Build history of the part. All positions in model axes, mm. Face numbers are marked on the shaded views. A direction names the side the tool comes from. Round coordinates to 2 decimals unless told otherwise and drop trailing zeros. Loops run counter-clockwise (first coordinate to the right, second up) from the corner with the lowest first, then second, coordinate; pieces in that order, holes last. Notation, with made-up numbers: (-34.5, 64.5) - (-30.5, 64.5) arc R33 cw to (-30.5, 96.5) - close; hole circle Ø7 at (37, 87.5). An arc over 180 degrees is marked (long way). Use one line per item in the form item = value. Start each with the question number.
Q1. Saw through at C-C (x = 4.25). Give the cut face in (y, z).
Q2. Drill centre lines: line 1 (Y direction, x = -1.1, z = 12.3); line 2 (X direction, y = 2, z = 5.5); line 3 (X direction, y = 4, z = -1.75). Where is each one in solid material? Low to high.
Q3. Pin check, flat tips, straight feed: pin 1 (3 mm diameter, centred on x = -1.1, y = 5, fed in from +Z); pin 2 (1.2 mm diameter, centred on x = -1.1, y = 11.75, fed in from +Z); pin 3 (2 mm diameter, centred on x = -9, z = 1.5, fed in from +Y). Stop position of each tip, or through.
Q4. 3-axis set-ups, long thin cutter, end or side, ignore diameter. For the marked faces 4 and 5: which of +Z, -Z, +X, -X, +Y, -Y reach the whole face in a straight line?
Q5. Saw through at B-B (z = 2.25). Give the cut face in (x, y).
Q6. Saw through at D-D (y = 5). Give the cut face in (x, z).
Q7. Saw through at A-A (y = 7). Give the cut face in (x, z).
Q8. Mould opens along Z. For the marked faces 1, 2 and 3 say: released by +Z, released by -Z, zero draft, split by the parting line, or undercut.
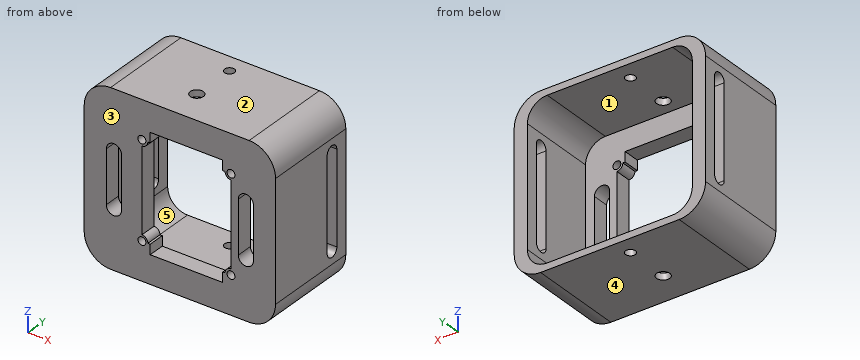
```python
from build123d import *

# Parameters (mm, degrees)
SKETCH1_W                = 25
SKETCH1_H                = 24
SKETCH1_R                = 0.6
BOSS_EXTRUDE1_DEPTH      = 2.5
CUT_EXTRUDE1_DEPTH       = 3.5
SKETCH8_W                = 11
SKETCH8_H                = 17.5
CUT_EXTRUDE4_DEPTH       = 3.5
SKETCH2_W                = 29
SKETCH2_H                = 26
SKETCH2_W_2              = 25
SKETCH2_H_2              = 24
BOSS_EXTRUDE2_DEPTH      = 12
BOSS_EXTRUDE2_DEPTH_BACK = 2.5
SKETCH5_R                = 0.75
SKETCH5_R_2              = 1
CUT_EXTRUDE2_DEPTH       = 26
CUT_EXTRUDE2_DEPTH_BACK  = 2
FILLET1_R                = 3
FILLET2_R                = 4
CUT_EXTRUDE5_DEPTH       = 30


with BuildPart() as part:
    # Sketch1 → Boss-Extrude1 (new body)
    with BuildSketch(Plane(origin=(0, 0, 0), x_dir=(1, 0, 0), z_dir=(0, 1, 0))):
        Rectangle(SKETCH1_W, SKETCH1_H)
        with Locations((7.75, 7.25)):
            Circle(SKETCH1_R, mode=Mode.SUBTRACT)
        with Locations((7.75, -7.25)):
            Circle(SKETCH1_R, mode=Mode.SUBTRACT)
        with Locations((-5.75, -7.25)):
            Circle(SKETCH1_R, mode=Mode.SUBTRACT)
        with Locations((-5.75, 7.25)):
            Circle(SKETCH1_R, mode=Mode.SUBTRACT)
        with BuildLine():
            Line((8.85, -4), (8.85, 4))
            ThreePointArc((8.85, 4), (10, 5.15), (11.15, 4))
            Line((11.15, 4), (11.15, -4))
            ThreePointArc((11.15, -4), (10, -5.15), (8.85, -4))
        make_face(mode=Mode.SUBTRACT)
        with BuildLine():
            Line((-8.85, -4), (-8.85, 4))
            ThreePointArc((-8.85, 4), (-10, 5.15), (-11.15, 4))
            Line((-11.15, 4), (-11.15, -4))
            ThreePointArc((-11.15, -4), (-10, -5.15), (-8.85, -4))
        make_face(mode=Mode.SUBTRACT)
    extrude(amount=BOSS_EXTRUDE1_DEPTH)

    # Sketch3 → Cut-Extrude1 (cut, through all)
    with BuildSketch(Plane(origin=(0, 2.5, 0), x_dir=(1, 0, 0), z_dir=(0, 1, 0))):
        with BuildLine():
            Line((-4.85, 7.25), (6.85, 7.25))
            ThreePointArc((6.85, 7.25), (7.113603897, 6.613603897), (7.75, 6.35))
            Line((7.75, 6.35), (7.75, -6.35))
            ThreePointArc((7.75, -6.35), (7.113603897, -6.613603897), (6.85, -7.25))
            Line((6.85, -7.25), (-4.85, -7.25))
            ThreePointArc((-4.85, -7.25), (-5.113603897, -6.613603897), (-5.75, -6.35))
            Line((-5.75, -6.35), (-5.75, 6.35))
            ThreePointArc((-5.75, 6.35), (-5.113603897, 6.613603897), (-4.85, 7.25))
        make_face()
    extrude(amount=-CUT_EXTRUDE1_DEPTH, mode=Mode.SUBTRACT)

    # Sketch8 → Cut-Extrude4 (cut, through all)
    with BuildSketch(Plane(origin=(0, 2.5, 0), x_dir=(1, 0, 0), z_dir=(0, 1, 0))):
        with Locations((1, 0)):
            Rectangle(SKETCH8_W, SKETCH8_H)
    extrude(amount=-CUT_EXTRUDE4_DEPTH, mode=Mode.SUBTRACT)

    # Sketch2 → Boss-Extrude2 (add, two sides)
    with BuildSketch(Plane(origin=(0, 2.5, 0), x_dir=(1, 0, 0), z_dir=(0, 1, 0))) as boss_extrude2_sk:
        Rectangle(SKETCH2_W, SKETCH2_H)
        Rectangle(SKETCH2_W_2, SKETCH2_H_2, mode=Mode.SUBTRACT)
    extrude(amount=BOSS_EXTRUDE2_DEPTH)
    extrude(boss_extrude2_sk.sketch, amount=-BOSS_EXTRUDE2_DEPTH_BACK)

    # Sketch5 → Cut-Extrude2 (cut, two sides)
    with BuildSketch(Plane.XY.offset(-12)) as cut_extrude2_sk:
        with Locations((-1.1, 11.75)):
            Circle(SKETCH5_R)
        with Locations((-1.1, 5)):
            Circle(SKETCH5_R_2)
    extrude(amount=CUT_EXTRUDE2_DEPTH, mode=Mode.SUBTRACT)
    extrude(cut_extrude2_sk.sketch, amount=-CUT_EXTRUDE2_DEPTH_BACK, mode=Mode.SUBTRACT)

    # Fillet1
    fillet1_edges = [part.edges().sort_by_distance(p)[0] for p in [
        (12.5, 8.5, 12),
        (-12.5, 8.5, -12),
        (12.5, 8.5, -12),
        (-12.5, 8.5, 12),
    ]]
    fillet(fillet1_edges, radius=FILLET1_R)

    # Fillet2
    fillet2_edges = [part.edges().sort_by_distance(p)[0] for p in [
        (-14.5, 7.25, 13),
        (14.5, 7.25, 13),
        (14.5, 7.25, -13),
        (-14.5, 7.25, -13),
    ]]
    fillet(fillet2_edges, radius=FILLET2_R)

    # Sketch9 → Cut-Extrude5 (cut, through all)
    with BuildSketch(Plane(origin=(14.5, 0, 0), x_dir=(0, 0, -1), z_dir=(1, 0, 0))):
        with BuildLine():
            Line((-7, 12.65), (7, 12.65))
            ThreePointArc((7, 12.65), (8, 11.65), (7, 10.65))
            Line((7, 10.65), (-7, 10.65))
            ThreePointArc((-7, 10.65), (-8, 11.65), (-7, 12.65))
        make_face()
    extrude(amount=-CUT_EXTRUDE5_DEPTH, mode=Mode.SUBTRACT)


solid = part.part
```
Report:
q1.outline = (0, -13) - (14.5, -13) - (14.5, -12) - (2.5, -12) - (2.5, -8.75) - (0, -8.75) - close; (0, 8.75) - (2.5, 8.75) - (2.5, 12) - (14.5, 12) - (14.5, 13) - (0, 13) - close
q2.line_1 = 0 to 4, 6 to 11, 12.5 to 14.5
q2.line_2 = -14.5 to -5.75, 7.75 to 14.5
q2.line_3 = -14.5 to -12.5, 12.5 to 14.5
q3.pin_1 = 13
q3.pin_2 = through
q3.pin_3 = 2.5
q4.face_4 = -Z, +X, -X, +Y, -Y
q4.face_5 = +Y
q5.outline = (-14.5, 0) - (-11.15, 0) - (-11.15, 2.5) - (-12.5, 2.5) - (-12.5, 10.65) - (-14.5, 10.65) - close; (-14.5, 12.65) - (-12.5, 12.65) - (-12.5, 14.5) - (-14.5, 14.5) - close; (-8.85, 0) - (-5.75, 0) - (-5.75, 2.5) - (-8.85, 2.5) - close; (7.75, 0) - (8.85, 0) - (8.85, 2.5) - (7.75, 2.5) - close; (11.15, 0) - (14.5, 0) - (14.5, 10.65) - (12.5, 10.65) - (12.5, 2.5) - (11.15, 2.5) - close; (12.5, 12.65) - (14.5, 12.65) - (14.5, 14.5) - (12.5, 14.5) - close
q6.outline = (-14.5, -9) arc R4 ccw to (-10.5, -13) - (-2.1, -13) - (-2.1, -12) - (-9.5, -12) arc R3 cw to (-12.5, -9) - (-12.5, 9) arc R3 cw to (-9.5, 12) - (-2.1, 12) - (-2.1, 13) - (-10.5, 13) arc R4 ccw to (-14.5, 9) - close; (-0.1, -13) - (10.5, -13) arc R4 ccw to (14.5, -9) - (14.5, 9) arc R4 ccw to (10.5, 13) - (-0.1, 13) - (-0.1, 12) - (9.5, 12) arc R3 cw to (12.5, 9) - (12.5, -9) arc R3 cw to (9.5, -12) - (-0.1, -12) - close
q7.outline = (-14.5, -9) arc R4 ccw to (-10.5, -13) - (10.5, -13) arc R4 ccw to (14.5, -9) - (14.5, 9) arc R4 ccw to (10.5, 13) - (-10.5, 13) arc R4 ccw to (-14.5, 9) - close; hole (-12.5, -9) arc R3 ccw to (-9.5, -12) - (9.5, -12) arc R3 ccw to (12.5, -9) - (12.5, 9) arc R3 ccw to (9.5, 12) - (-9.5, 12) arc R3 ccw to (-12.5, 9) - close
q8.face_1 = undercut
q8.face_2 = released by +Z
q8.face_3 = zero draft
